The drawing under review shows one solid part. Ordinate dimensions are in mm from its lowest x, y, z. A direction names the side the tool comes from. Round coordinates to 2 decimals unless told otherwise and drop trailing zeros. Order: outer loops, then holes, each group sorted by start corner. A loop starts at its lowest first (then second) coordinate and runs counter-clockwise, first axis right, second up.
1) Mouldability with a two-part tool opening along Z and no side actions: class the marked faces 1, 2 and 3 as pulls with the +Z half, pulls with the -Z half, needs draft (parallel to the pull), parting line crosses it, or undercut.
2) Machinability: for the marked faces 4 and 5, which of the approach directions +Z, -Z, +X, -X, +Y, -Y give a long, thin tool a straight path to every point of the face, cutting with its end or side? Answer none if there is none.
3) Consider section A-A (x = 163.5). Give the boundary of the cut face in (y, z).
4) To check wall thickness, follow L1, parallel to Y at x = 21, z = 310; L2, parallel to Z at x = 192.5, y = 127; L3, parallel to X at y = 163, z = 186.5. State the ranges of each line that lie inside material, in increasing order.
5) Consider section D-D (z = 208). Give the boundary of the cut face in (x, y), then the cut area to 3 significant figures.
6) Consider section C-C (z = 158). Give the boundary of the cut face in (x, y), then the cut area to 3 significant figures.
7) Clearance check with flat-ended pins moving along their axes: P1, Ø24.5, axis at y = 165, z = 208, coming from the -X side; P2, Ø18, axis at x = 21, y = 175, coming from the +Z side. State where each tip first meets the part, or that it passes through.
8) Consider section B-B (y = 115). Give the boundary of the cut face in (x, z), then the cut area to 3 significant figures.
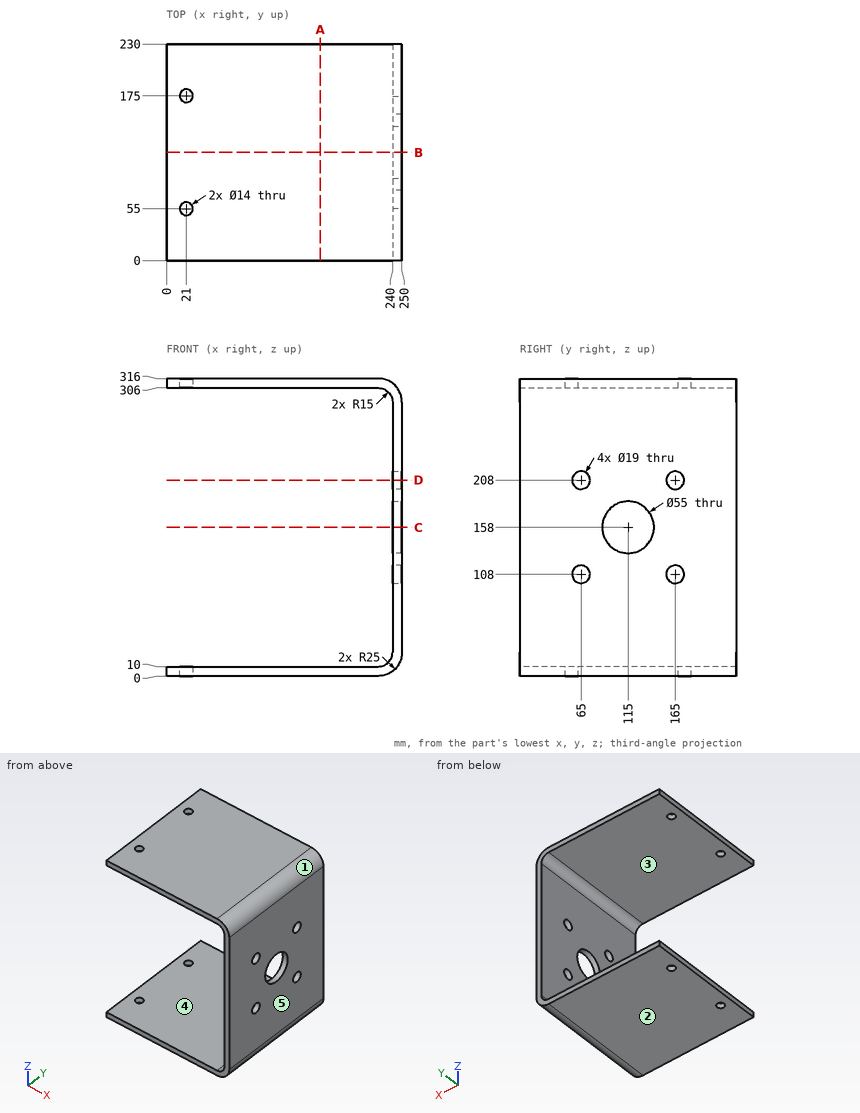
Answer below:
1. face 1: pulls with the +Z half
1. face 2: pulls with the -Z half
1. face 3: undercut
2. face 4: -X, +Y, -Y
2. face 5: +Z, -Z, +X, +Y, -Y
3. outline: (0, 0) - (230, 0) - (230, 10) - (0, 10) - close; (0, 306) - (230, 306) - (230, 316) - (0, 316) - close
4. L1: y = 0 to 48, 62 to 168, 182 to 230
4. L2: z = 0 to 10, 306 to 316
4. L3: x = 240 to 250
5. outline: (240, 0) - (250, 0) - (250, 55.5) - (240, 55.5) - close; (240, 74.5) - (250, 74.5) - (250, 155.5) - (240, 155.5) - close; (240, 174.5) - (250, 174.5) - (250, 230) - (240, 230) - close
5. area: 1,920 mm2
6. outline: (240, 0) - (250, 0) - (250, 87.5) - (240, 87.5) - close; (240, 142.5) - (250, 142.5) - (250, 230) - (240, 230) - close
6. area: 1,750 mm2
7. P1: stops at x = 240
7. P2: stops at z = 316
8. outline: (0, 0) - (225, 0) arc R25 ccw to (250, 25) - (250, 130.5) - (240, 130.5) - (240, 25) arc R15 cw to (225, 10) - (0, 10) - close; (0, 306) - (225, 306) arc R15 cw to (240, 291) - (240, 185.5) - (250, 185.5) - (250, 291) arc R25 ccw to (225, 316) - (0, 316) - close
8. area: 7,240 mm2
